Model file for the job. Use its own axes, mm. A direction names the side the tool comes from. Coordinates: 2 decimals unless noted, no trailing zeros. Write each loop counter-clockwise with the first axis right and the second up, starting at its lowest first coordinate (ties: lowest second). Pieces come first, ordered by that corner, then holes. Notation, with made-up numbers: M 72.5,2 L 83.5,2 A21 ccw 83.5,12 Z; hole C -16,81.25 d8. An arc over 180 degrees is marked long. One line per question, with ' | ' between items. Start each with the question number.
(1) Cut at C-C (z = 1). Write the cut outline in (x, y).
(2) Tool access for faces 1 (the face through (-16, -17.3, 4.7)), 2 (the face through (0, -23, 3.2)), 3 (the face through (24, 1, 4.7)): list every direction of +Z, -Z, +X, -X, +Y, -Y with a clear straight run to the whole face (end or side of a thin tool).
(3) Cut at D-D (z = 6.5). Write the cut outline in (x, y).
(4) Flat gauge pins, fed straight in: pin 1 Ø1.2 at (x, y) = (23.5, 0) entering from +Z; pin 2 Ø3 at (x, z) = (-6.5, 2) entering from +Y; pin 3 Ø2.5 at (x, y) = (-23, 0.5) entering from +Z; pin 4 Ø1.5 at (x, z) = (17, 7) entering from +Y. Where does each tip first touch, or does it go through?
(5) Cut at A-A (x = 6). Write the cut outline in (y, z).
(6) Two-plate mould, pull along X, no slides. Class faces 4 (the face through (-17.212, -17.073, 3.96)), 5 (the face through (-1, 23, 4.7)), 6 (the face through (-0.163, 22.768, 3.96)): +X half, -X half, draft (parallel to the pull), parting line (faces both ways), or undercut.
(7) Wall check: probe 1 along Z at (x, y) = (12, 6); probe 2 along X at (y, z) = (-4.5, 3.75); probe 3 along Y at (x, z) = (-16, 2.25). Give the ranges that are in metal, low to high.
(8) Cut at B-B (y = -14). Write the cut outline in (x, z), plus the area to 3 significant figures.
from build123d import *

# Parameters (mm, degrees)
F0_R     = 25
F0_R_2   = 3
F1_DEPTH = 2
F2_R     = 19.3
F2_R_2   = 17.3
F3_DEPTH = 3
F4_R     = 1.5
F5_DEPTH = 2.7
F6_R     = 5
F6_R_2   = 3
F7_DEPTH = 6
F8_R     = 0.75
F9_DEPTH = 1.5


with BuildPart() as f1:
    # F0 (on Top) → F1 (new body)
    with BuildSketch(Plane.XY):
        Circle(F0_R)
        Circle(F0_R_2, mode=Mode.SUBTRACT)
    extrude(amount=F1_DEPTH)

    # F2 (on face) → F3 (join)
    with BuildSketch(Plane.XY.offset(2)):
        Circle(F2_R)
        Circle(F2_R_2, mode=Mode.SUBTRACT)
    extrude(amount=F3_DEPTH)

    # F4 (on face) → F5 (join)
    with BuildSketch(Plane.XY.offset(2)):
        with Locations((0, 23.5)):
            Circle(F4_R)
        with Locations((-16.617009, 16.617009)):
            Circle(F4_R)
        with Locations((-23.5, 0)):
            Circle(F4_R)
        with Locations((-16.617009, -16.617009)):
            Circle(F4_R)
        with Locations((0, -23.5)):
            Circle(F4_R)
        with Locations((16.617009, -16.617009)):
            Circle(F4_R)
        with Locations((23.5, 0)):
            Circle(F4_R)
        with Locations((16.617009, 16.617009)):
            Circle(F4_R)
    extrude(amount=F5_DEPTH)

    # F6 (on face) → F7 (join)
    with BuildSketch(Plane.XY.offset(2)):
        Circle(F6_R)
        Circle(F6_R_2, mode=Mode.SUBTRACT)
    extrude(amount=F7_DEPTH)

    # F8 (on face) → F9 (cut)
    with BuildSketch(Plane.XY.offset(4.7)):
        with Locations((23.5, 0)):
            Circle(F8_R)
        with Locations((16.617009, 16.617009)):
            Circle(F8_R)
        with Locations((0, 23.5)):
            Circle(F8_R)
        with Locations((-16.617009, 16.617009)):
            Circle(F8_R)
        with Locations((-23.5, 0)):
            Circle(F8_R)
        with Locations((-16.617009, -16.617009)):
            Circle(F8_R)
        with Locations((0, -23.5)):
            Circle(F8_R)
        with Locations((16.617009, -16.617009)):
            Circle(F8_R)
    extrude(amount=-F9_DEPTH, mode=Mode.SUBTRACT)


solid = f1.part
Filled in:
1) outline: C 0,0 d50; hole C 0,0 d6
2) face 1: +Z, -X, -Y | face 2: +Z | face 3: +Z, +X, +Y, -Y
3) outline: C 0,0 d10; hole C 0,0 d6
4) pin 1: z = 3.2 | pin 2: y = 24.49 | pin 3: z = 4.7 | pin 4: through
5) outline: M -24.27,0 L 24.27,0 L 24.27,2 L 18.34,2 L 18.34,5 L 16.23,5 L 16.23,2 L -16.23,2 L -16.23,5 L -18.34,5 L -18.34,2 L -24.27,2 Z
6) face 4: undercut | face 5: draft | face 6: undercut
7) probe 1: 0 to 2 | probe 2: -18.77 to -16.7, -2.18 to 2.18, 16.7 to 18.77 | probe 3: -17.98 to -15.25, -10.79 to -6.58, 6.58 to 10.79, 15.25 to 17.98
8) outline: M -20.71,0 L 20.71,0 L 20.71,2 L 13.28,2 L 13.28,5 L 10.16,5 L 10.16,2 L -10.16,2 L -10.16,5 L -13.28,5 L -13.28,2 L -20.71,2 Z | area: 102 mm²
